from build123d import *

# Parameters (mm, degrees)
EXTRUDE_1_DEPTH     = 5
SKETCH_2_R          = 1.65
CUT_EXTRUDE_1_DEPTH = 10


with BuildPart() as part:
    # 草图1 → 凸台-拉伸1 (new body)
    with BuildSketch(Plane(origin=(0, 0, 0), x_dir=(0, 0, -1), z_dir=(1, 0, 0))):
        with BuildLine():
            ThreePointArc((20, -8), (16, -4), (20, 0))
            Line((20, 0), (0, 0))
            Line((0, 0), (0, -8))
            Line((0, -8), (20, -8))
        make_face()
        with BuildLine():
            Line((20, -8), (20, 0))
            ThreePointArc((20, 0), (16, -4), (20, -8))
        make_face()
        with BuildLine():
            Line((23.464101615, -6), (20, 0))
            Line((20, 0), (20, -8))
            ThreePointArc((20, -8), (22, -7.464101615), (23.464101615, -6))
        make_face()
        with BuildLine():
            ThreePointArc((24, -4), (22.828427125, -1.171572875), (20, 0))
            Line((20, 0), (23.464101615, -6))
            ThreePointArc((23.464101615, -6), (23.863703305, -5.03527618), (24, -4))
        make_face()
        with BuildLine():
            Line((30, -17.320508076), (23.464101615, -6))
            ThreePointArc((23.464101615, -6), (22, -7.464101615), (20, -8))
            Line((20, -8), (26.535898385, -19.320508076))
            ThreePointArc((26.535898385, -19.320508076), (28, -17.856406461), (30, -17.320508076))
        make_face()
        with BuildLine():
            ThreePointArc((34, -21.320508076), (32.828427125, -18.492080951), (30, -17.320508076))
            Line((30, -17.320508076), (30, -25.320508076))
            ThreePointArc((30, -25.320508076), (32.828427125, -24.1489352), (34, -21.320508076))
        make_face()
        with BuildLine():
            Line((30, -25.320508076), (30, -17.320508076))
            ThreePointArc((30, -17.320508076), (28, -17.856406461), (26.535898385, -19.320508076))
            Line((26.535898385, -19.320508076), (30, -25.320508076))
        make_face()
        with BuildLine():
            Line((30, -25.320508076), (26.535898385, -19.320508076))
            ThreePointArc((26.535898385, -19.320508076), (26.535898385, -23.320508076), (30, -25.320508076))
        make_face()
    extrude(amount=EXTRUDE_1_DEPTH)

    # 草图2 → 切除-拉伸1 (cut)
    with BuildSketch(Plane(origin=(5, 0, 0), x_dir=(0, 0, -1), z_dir=(1, 0, 0))):
        with Locations((5, -4)):
            Circle(SKETCH_2_R)
        with Locations((30, -21.320508076)):
            Circle(SKETCH_2_R)
    extrude(amount=-CUT_EXTRUDE_1_DEPTH, mode=Mode.SUBTRACT)


solid = part.part
Could you check a few things on this model? Use its own coordinates, in mm. A direction names the side the tool comes from. Give positions to 0.01 mm unless a question says otherwise; leave off trailing zeros. Write each loop counter-clockwise with the first axis right and the second up, starting at its lowest first coordinate (ties: lowest second). Pieces come first, ordered by that corner, then holes. Notation, with made-up numbers: (-12.75, 33) -> (3.25, 33) arc R5 ccw to (3.25, 39) -> close; hole circle Ø9 at (84, 87). An arc over 180 degrees is marked (long way). Answer as CSV lines item,"result". Start each with the question number.
(1) If we section it at A-A, the plane x = 1.5: Write out the boundary of the cut face in (y, z), and give its area (3 significant figures).
(2) If we section it at B-B, the plane z = -5: Write out the boundary of the cut face in (x, y), and give its area (3 significant figures).
(3) If we section it at C-C, the plane y = -3.25: Write out the boundary of the cut face in (x, z), and give its area (3 significant figures).
(4) I'm going to push flat-ended pins straight in: pin 1 Ø2 at (x, y) = (3, -20) entering from -Z; pin 2 Ø4.5 at (y, z) = (-4, -5) entering from -X; pin 3 Ø1.5 at (x, y) = (1, -18) entering from +Z; pin 4 Ø1 at (x, z) = (3.5, -3.5) entering from -Y. Where does each tip first touch, or does it pass through?
(5) Please list where these lines run through material, in increasing order: line 1 (Z direction, x = 3.05, y = -3.75); line 2 (Y direction, x = 3.6, z = -13.5); line 3 (Z direction, x = 3.6, y = -2).
(6) Which directions (+Z, -Z, +X, -X, +Y, -Y) give clear straight access to the entire face, cutting with the end or side of a thin tool? Please do faces 1 (the face through (2.54, -22.93, -29.64)), 2 (the face through (2, -8, -10)).
(7) If we mould it in two halves opening along Z, with no side actions, what happens to faces 3 (the face through (5, -7, -16)), 4 (the face through (2.46, -11.74, -26.78)), 5 (the face through (2.54, -5, -3.69))? For each: +Z half, -Z half, draft (parallel to the pull), parting line (faces both ways), or undercut.
(8) If we section it at D-D, the plane y = -7.5: Write out the boundary of the cut face in (x, z).
Answer list:
1,outline,"(-19.32, -26.54) arc R4 ccw (long way) to (-17.32, -30) -> (-6, -23.46) arc R4 ccw to (0, -20) -> (0, 0) -> (-8, 0) -> (-8, -20) -> close; hole circle Ø3.3 at (-21.32, -30); hole circle Ø3.3 at (-4, -5)"
1,area,"268 mm^2"
2,outline,"(0, -8) -> (5, -8) -> (5, -5.65) -> (0, -5.65) -> close; (0, -2.35) -> (5, -2.35) -> (5, 0) -> (0, 0) -> close"
2,area,"23.5 mm^2"
3,outline,"(0, -23.93) -> (5, -23.93) -> (5, -6.47) -> (0, -6.47) -> close; (0, -3.53) -> (5, -3.53) -> (5, 0) -> (0, 0) -> close"
3,area,"105 mm^2"
4,pin 1,"z = -33.99"
4,pin 2,"x = 0"
4,pin 3,"z = -25.34"
4,pin 4,"y = -8"
5,line 1,"-23.99 to -6.63, -3.37 to 0"
5,line 2,"-8 to 0"
5,line 3,"-23.46 to 0"
6,face 1,"+X, -X"
6,face 2,"+Z, +X, -X, -Y"
7,face 3,"draft"
7,face 4,"-Z half"
7,face 5,"undercut"
8,outline,"(0, -24.33) -> (5, -24.33) -> (5, 0) -> (0, 0) -> close"
